Build history of the part. All positions in model axes, mm. A direction names the side the tool comes from. Round coordinates to 2 decimals unless told otherwise and drop trailing zeros. Order: outer loops, then holes, each group sorted by start corner. A loop starts at its lowest first (then second) coordinate and runs counter-clockwise, first axis right, second up. Notation, with made-up numbers: (87, -3.75) - (113, -3.75) arc R8 cw to (113, 3.25) - close; hole circle Ø3 at (15, 22). An arc over 180 degrees is marked (long way). Write each question's results on one line, items separated by ' | '. Start each with the question number.
```python
from build123d import *

# Parameters (mm, degrees)
SKETCH1_R           = 12.7
BOSS_EXTRUDE1_DEPTH = 25.4
SKETCH2_R           = 2.921
BOSS_EXTRUDE2_DEPTH = 3.175
SKETCH4_R           = 1.2065
CUT_EXTRUDE1_DEPTH  = 7.62
SKETCH6_R           = 0.9525
BOSS_EXTRUDE3_DEPTH = 6.35


with BuildPart() as part:
    # Sketch1 → Boss-Extrude1 (new body)
    with BuildSketch(Plane.XY):
        Circle(SKETCH1_R)
    extrude(amount=BOSS_EXTRUDE1_DEPTH)

    # Sketch2 → Boss-Extrude2 (add)
    with BuildSketch(Plane.XY.offset(25.4)):
        Circle(SKETCH2_R)
    extrude(amount=BOSS_EXTRUDE2_DEPTH)

    # Sketch4 → Cut-Extrude1 (cut)
    with BuildSketch(Plane.XY.offset(25.4)):
        with Locations((-5.7785, 0)):
            Circle(SKETCH4_R)
        with Locations((5.7785, 0)):
            Circle(SKETCH4_R)
    extrude(amount=-CUT_EXTRUDE1_DEPTH, mode=Mode.SUBTRACT)

    # Sketch6 → Boss-Extrude3 (add)
    with BuildSketch(Plane.XY.offset(28.575)):
        Circle(SKETCH6_R)
    extrude(amount=BOSS_EXTRUDE3_DEPTH)


solid = part.part
```
1. Cut at D-D (z = 7.5). List the corners of the cut face in (x, y), plus the area to 3 significant figures.
2. Mould opens along X. For faces 3 (the face through (-0.21, -0.93, 31.71)), 4 (the face through (0, 0, 0)), 5 (the face through (-4.628, 0.362, 21.643)) say: pulls with the +X half, pulls with the -X half, needs draft (parallel to the pull), parting line crosses it, or undercut.
3. 3-axis set-ups, long thin cutter, end or side, ignore diameter. For faces 1 (the face through (0, 0, 34.925)), 2 (the face through (-0.633, -2.852, 26.965)): which of +Z, -Z, +X, -X, +Y, -Y reach the whole face in a straight line?
4. Cut at C-C (z = 27). List the corners of the cut face in (x, y), plus the area to 3 significant figures.
5. Cut at A-A (x = 0). List the corners of the cut face in (y, z) (1 decimal).
6. Wall check: line 1 (Z direction, x = -4, y = -6.25); line 2 (Y direction, x = 6, z = 24); line 3 (Y direction, x = -5.75, z = 20.5). Give the ranges that are in metal, low to high. Write a range as from..to.
7. Flat gauge pins, fed straight in: pin 1 Ø2 at (x, y) = (-5.78, 0) entering from +Z; pin 2 Ø10 at (y, z) = (5.5, 17.5) entering from +X; pin 3 Ø12 at (x, z) = (9.5, 23.5) entering from +Y. Where does each tip first touch, or does it go through?
8. Cut at B-B (y = 0). List the corners of the cut face in (x, z) (1 decimal).
A:
1) outline: circle Ø25.4 at (0, 0) | area: 507 mm^2
2) face 3: parting line crosses it | face 4: needs draft | face 5: undercut
3) face 1: +Z, +X, -X, +Y, -Y | face 2: +Z
4) outline: circle Ø5.84 at (0, 0) | area: 26.8 mm^2
5) outline: (-12.7, 0) - (12.7, 0) - (12.7, 25.4) - (2.9, 25.4) - (2.9, 28.6) - (1, 28.6) - (1, 34.9) - (-1, 34.9) - (-1, 28.6) - (-2.9, 28.6) - (-2.9, 25.4) - (-12.7, 25.4) - close
6) line 1: z = 0..25.4 | line 2: y = -11.19..-1.19, 1.19..11.19 | line 3: y = -11.32..-1.21, 1.21..11.32
7) pin 1: stops at z = 17.78 | pin 2: stops at x = 12.69 | pin 3: stops at y = 12.21
8) outline: (-12.7, 0) - (12.7, 0) - (12.7, 25.4) - (7, 25.4) - (7, 17.8) - (4.6, 17.8) - (4.6, 25.4) - (2.9, 25.4) - (2.9, 28.6) - (1, 28.6) - (1, 34.9) - (-1, 34.9) - (-1, 28.6) - (-2.9, 28.6) - (-2.9, 25.4) - (-4.6, 25.4) - (-4.6, 17.8) - (-7, 17.8) - (-7, 25.4) - (-12.7, 25.4) - close
